Here's the drawing with two shaded views (mm, measured from the low corner). I have some questions. A direction names the side the tool comes from. Round coordinates to 2 decimals unless told otherwise and drop trailing zeros. Order: outer loops, then holes, each group sorted by start corner. A loop starts at its lowest first (then second) coordinate and runs counter-clockwise, first axis right, second up.
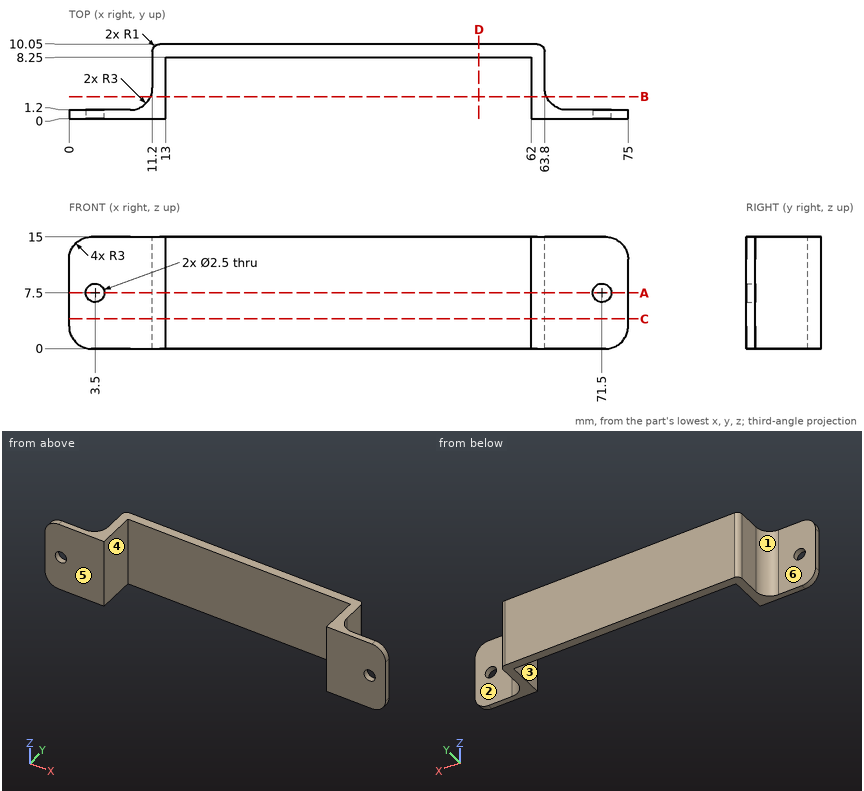
Q1. I need wall thicknesses on L1, parallel to Z at x = 71.5, y = 0.7; L2, parallel to X at y = 6, z = 7; L3, parallel to Y at x = 70.5, z = 4.5. Which ranges of each line are inside material? Lowest first, please.
Q2. Imagine slicing it at B-B, the plane y = 3. Please give me the cut outline in (x, z), then the cut area to 3 significant figures.
Q3. We'd pull the mould along X, two halves only. Please class the marked faces 1, 2 and 3: released by +X, released by -X, zero draft, split by the parting line, or undercut.
Q4. For the marked faces 4, 5 and 6, which set-ups out of +Z, -Z, +X, -X, +Y, -Y let a thin tool reach every point of the face, with its end or its side?
Q5. Imagine slicing it at D-D, the plane x = 55. Please give me the cut outline in (y, z), then the cut area to 3 significant figures.
Q6. Imagine slicing it at A-A, the plane z = 7.5. Please give me the cut outline in (x, y).
Q7. For P1, Ø8, axis at x = 50.5, z = 3, coming from the -Y side; P2, Ø6.5, axis at x = 2.5, z = 8, coming from the +Y side; P3, Ø4, axis at x = 37.5, y = 5, coming from the -Z side; P4, Ø1, axis at y = 1.5, z = 2.5, coming from the +X side, each with a flat end and sliding along its axis, tell me the tip position at first contact or that it passes through.
Q8. Imagine slicing it at C-C, the plane z = 4. Please give me the cut outline in (x, y), then the cut area to 3 significant figures.
Filled in:
1. L1: z = 0 to 6.25, 8.75 to 15
1. L2: x = 11.2 to 13, 62 to 63.8
1. L3: y = 0 to 1.2
2. outline: (10.95, 0) - (13, 0) - (13, 15) - (10.95, 15) - close; (62, 0) - (64.05, 0) - (64.05, 15) - (62, 15) - close
2. area: 61.5 mm2
3. face 1: released by -X
3. face 2: zero draft
3. face 3: undercut
4. face 4: +Z, -Z, -Y
4. face 5: +Z, -Z, +X, -X, -Y
4. face 6: +Z, -Z, -X, +Y
5. outline: (8.25, 0) - (10.05, 0) - (10.05, 15) - (8.25, 15) - close
5. area: 27.0 mm2
6. outline: (0, 0) - (2.25, 0) - (2.25, 1.2) - (0, 1.2) - close; (4.75, 0) - (13, 0) - (13, 8.25) - (62, 8.25) - (62, 0) - (70.25, 0) - (70.25, 1.2) - (66.8, 1.2) arc R3 cw to (63.8, 4.2) - (63.8, 9.05) arc R1 ccw to (62.8, 10.05) - (12.2, 10.05) arc R1 ccw to (11.2, 9.05) - (11.2, 4.2) arc R3 cw to (8.2, 1.2) - (4.75, 1.2) - close; (72.75, 0) - (75, 0) - (75, 1.2) - (72.75, 1.2) - close
7. P1: stops at y = 8.25
7. P2: stops at y = 1.2
7. P3: passes through
7. P4: stops at x = 75
8. outline: (0, 0) - (13, 0) - (13, 8.25) - (62, 8.25) - (62, 0) - (75, 0) - (75, 1.2) - (66.8, 1.2) arc R3 cw to (63.8, 4.2) - (63.8, 9.05) arc R1 ccw to (62.8, 10.05) - (12.2, 10.05) arc R1 ccw to (11.2, 9.05) - (11.2, 4.2) arc R3 cw to (8.2, 1.2) - (0, 1.2) - close
8. area: 155 mm2
